from build123d import *

# Parameters (mm, degrees)
CUT_EXTRUDE_1_DEPTH = 4
FILLET_1_R          = 0.3
CHAMFER_1_SIZE      = 1.6
FILLET_2_R          = 1


with BuildPart() as part:
    # Эскиз1 → Повернуть1 (revolve)
    with BuildSketch(Plane.XY):
        Polygon((0, 0), (0, 6.824573519), (5.5, 10), (6, 10), (6, 3.95), (13, 3.95), (15.05, 6), (36, 6), (36, 0), align=None)
    revolve(axis=Axis((36, 0, 0), (-1, 0, 0)))

    # Эскиз2 → Вырез-Вытянуть1 (cut)
    with BuildSketch(Plane.ZY):
        Polygon((1.732050808, 3), (-1.732050808, 3), (-3.464101615, 0), (-1.732050808, -3), (1.732050808, -3), (3.464101615, 0), align=None)
    extrude(amount=-CUT_EXTRUDE_1_DEPTH, mode=Mode.SUBTRACT)

    # Скругление1
    fillet_1_edges = [part.edges().sort_by_distance(p)[0] for p in [
        (6, -10, 0),
    ]]
    fillet(fillet_1_edges, radius=FILLET_1_R)

    # Фаска1
    chamfer_1_edges = [part.edges().sort_by_distance(p)[0] for p in [
        (36, -6, 0),
    ]]
    chamfer(chamfer_1_edges, length=CHAMFER_1_SIZE)

    # Скругление2
    fillet_2_edges = [part.edges().sort_by_distance(p)[0] for p in [
        (6, -3.95, 0),
    ]]
    fillet(fillet_2_edges, radius=FILLET_2_R)


solid = part.part
Could you check a few things on this model? Use its own coordinates, in mm. A direction names the side the tool comes from. Coordinates: 2 decimals unless noted, no trailing zeros. Order: outer loops, then holes, each group sorted by start corner. A loop starts at its lowest first (then second) coordinate and runs counter-clockwise, first axis right, second up. Notation, with made-up numbers: (1, 32) - (39, 32) arc R24 cw to (39, 63) - close; hole circle Ø10 at (78, -34). An arc over 180 degrees is marked (long way). Answer in a Markdown table with one row per item. Add a question column.
(1) If we section it at B-B, the plane x = 10: Please give me the cut outline in (y, z), then the cut area to 3 significant figures.
(2) If we mould it in two halves opening along Z, with no side actions, what happens to faces 1 (the face through (2, 1.5, 2.6)), 2 (the face through (36, 0, 0)), 3 (the face through (0.344, -1.522, 6.856))? For each: released by +Z, released by -Z, zero draft, split by the parting line, or undercut.
(3) If we section it at C-C, the plane x = 27: Please give me the cut outline in (y, z).
(4) I need wall thicknesses on L1, parallel to X at y = 1, z = -5.5; L2, parallel to X at y = 0.25, z = 3; L3, parallel to X at y = 5, z = -3. Which ranges of each line are inside material? Lowest first, please.
(5) Will these pins go through, and if not, where does the flat tip stop? pin 1 (4 mm diameter, centred on x = 11, y = 2, fed in from -Z); pin 2 (1 mm diameter, centred on x = 18.5, y = 5.5, fed in from -Z); pin 3 (10 mm diameter, centred on x = 25, y = -4.5, fed in from -Z); pin 4 (10 mm diameter, centred on y = -1.5, z = -7.5, fed in from +X).
(6) On a 3-axis mill with a long thin cutter (end or side, diameter ignored), from which of +Z, -Z, +X, -X, +Y, -Y can I reach the whole of each face in a straight line? I mean faces 4 (the face through (2, 1.5, -2.6)), 5 (the face through (10.042, -3.135, 2.404)), 6 (the face through (25, -6, 0)). Say none if no direction works.
(7) If we section it at A-A, the plane z = 0: Please give me the cut outline in (x, y).
Results are:
| question | item | result |
|---|---|---|
| 1 | outline | circle Ø7.9 at (0, 0) |
| 1 | area | 49.0 mm2 |
| 2 | face 1 | undercut |
| 2 | face 2 | zero draft |
| 2 | face 3 | split by the parting line |
| 3 | outline | circle Ø12 at (0, 0) |
| 4 | L1 | x = 0 to 6, 14.64 to 34.81 |
| 4 | L2 | x = 4 to 36 |
| 4 | L3 | x = 0 to 6, 14.88 to 34.57 |
| 5 | pin 1 | stops at z = -3.95 |
| 5 | pin 2 | stops at z = -3.32 |
| 5 | pin 3 | stops at z = -6 |
| 5 | pin 4 | stops at x = 36 |
| 6 | face 4 | -X |
| 6 | face 5 | none |
| 6 | face 6 | +X |
| 7 | outline | (0, -6.82) - (5.5, -10) - (5.7, -10) arc R0.3 ccw to (6, -9.7) - (6, -4.95) arc R1 cw to (7, -3.95) - (13, -3.95) - (15.05, -6) - (34.4, -6) - (36, -4.4) - (36, 4.4) - (34.4, 6) - (15.05, 6) - (13, 3.95) - (7, 3.95) arc R1 cw to (6, 4.95) - (6, 9.7) arc R0.3 ccw to (5.7, 10) - (5.5, 10) - (0, 6.82) - (0, 3) - (4, 3) - (4, -3) - (0, -3) - close |
